Drawing for the job (mm, zero at the part's lowest x, y, z). A direction names the side the tool comes from. Round coordinates to 2 decimals unless told otherwise and drop trailing zeros. Write each loop counter-clockwise with the first axis right and the second up, starting at its lowest first coordinate (ties: lowest second). Pieces come first, ordered by that corner, then holes.
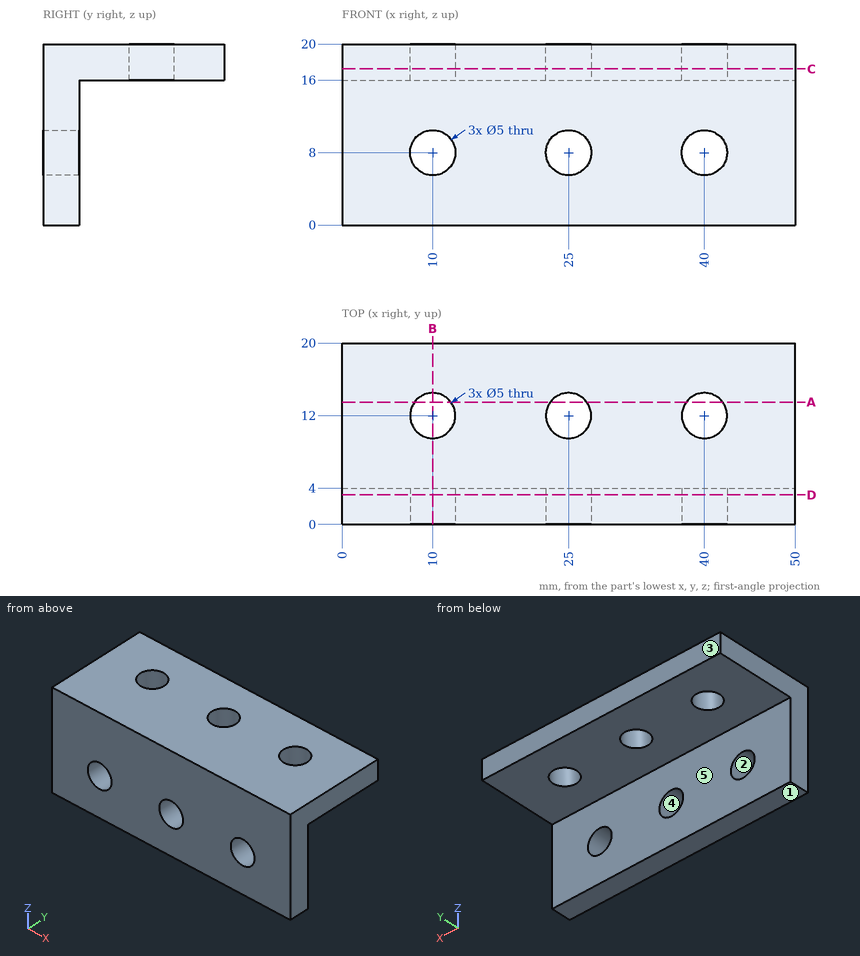
Q1. Saw through at A-A, the plane y = 13.5. Write the cut outline in (x, z).
Q2. Saw through at B-B, the plane x = 10. Write the cut outline in (y, z).
Q3. Saw through at C-C, the plane z = 17.25. Write the cut outline in (x, y), and give its area (3 significant figures).
Q4. Saw through at D-D, the plane y = 3.25. Write the cut outline in (x, z).
Q5. Tool access for the marked faces 4 and 5: list every direction of +Z, -Z, +X, -X, +Y, -Y with a clear straight run to the whole face (end or side of a thin tool).
Q6. Drop flat-ended pins along their axis: P1, Ø1, axis at x = 34, y = 11.5, coming from the -Z side; P2, Ø3, axis at x = 12.5, z = 10, coming from the +Y side. Give the stop position or say it passes through.
Q7. Wall check: line 1 (X direction, y = 3.05, z = 8); line 2 (Y direction, x = 25, z = 18); line 3 (X direction, y = 1.25, z = 6). Give the ranges that are in metal, low to high.
Q8. Two-plate mould, pull along Z, no slides. Class the marked faces 1, 2 and 3: released by +Z, released by -Z, zero draft, split by the parting line, or undercut.
Computed:
1. outline: (0, 16) - (8, 16) - (8, 20) - (0, 20) - close; (12, 16) - (23, 16) - (23, 20) - (12, 20) - close; (27, 16) - (38, 16) - (38, 20) - (27, 20) - close; (42, 16) - (50, 16) - (50, 20) - (42, 20) - close
2. outline: (0, 0) - (4, 0) - (4, 5.5) - (0, 5.5) - close; (0, 10.5) - (4, 10.5) - (4, 16) - (9.5, 16) - (9.5, 20) - (0, 20) - close; (14.5, 16) - (20, 16) - (20, 20) - (14.5, 20) - close
3. outline: (0, 0) - (50, 0) - (50, 20) - (0, 20) - close; hole circle Ø5 at (10, 12); hole circle Ø5 at (25, 12); hole circle Ø5 at (40, 12)
3. area: 941 mm2
4. outline: (0, 0) - (50, 0) - (50, 20) - (0, 20) - close; hole circle Ø5 at (10, 8); hole circle Ø5 at (25, 8); hole circle Ø5 at (40, 8)
5. face 4: +Y, -Y
5. face 5: -Z, +X, -X, +Y
6. P1: stops at z = 16
6. P2: stops at y = 4
7. line 1: x = 0 to 7.5, 12.5 to 22.5, 27.5 to 37.5, 42.5 to 50
7. line 2: y = 0 to 9.5, 14.5 to 20
7. line 3: x = 0 to 8.5, 11.5 to 23.5, 26.5 to 38.5, 41.5 to 50
8. face 1: released by -Z
8. face 2: undercut
8. face 3: zero draft
